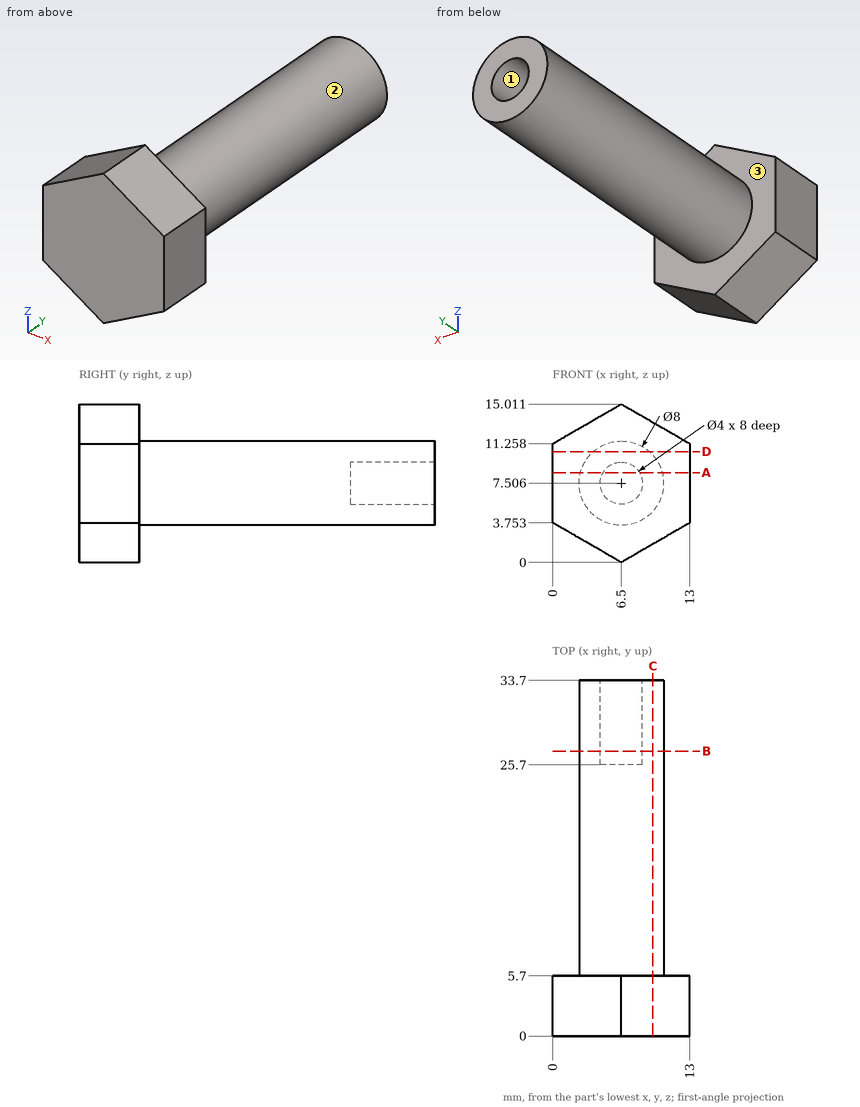
Could you check a few things on this drawing? It's one solid part, dimensions in mm from its lowest x, y, z. Coordinates: 2 decimals unless noted, no trailing zeros. Order: outer loops, then holes, each group sorted by start corner. A loop starts at its lowest first (then second) coordinate and runs counter-clockwise, first axis right, second up. Notation, with made-up numbers: (11.25, -32.5) - (26.25, -32.5) arc R23 ccw to (26.25, 0.5) - close; hole circle Ø9 at (56, -23.75). An arc over 180 degrees is marked (long way). Answer as a JSON object with one key per item and string values. Group by question number.
Q1. I need wall thicknesses on line 1 (X direction, y = 29.5, z = 7.5); line 2 (Y direction, x = 10.25, z = 10.25); line 3 (Z direction, x = 6.25, y = 23). Which ranges of each line are inside material? Lowest first, please. Write a range as from..to.
Q2. Imagine slicing it at A-A (z = 8.5). Please give me the cut outline in (x, y) (1 decimal).
Q3. Imagine slicing it at C-C (x = 9.5). Please give me the cut outline in (y, z), and give its area (3 significant figures).
Q4. Will these pins go through, and if not, where does the flat tip stop? P1, Ø1, axis at x = 3.5, y = 25, coming from the +Z side; P2, Ø1, axis at y = 13.5, z = 6.5, coming from the -X side; P3, Ø2, axis at x = 6, z = 8, coming from the +Y side.
Q5. Imagine slicing it at D-D (z = 10.5). Please give me the cut outline in (x, y), and give its area (3 significant figures).
Q6. Imagine slicing it at B-B (y = 27). Please give me the cut outline in (x, z) (1 decimal).
Q7. We'd pull the mould along Z, two halves only. Please class the marked faces 1, 2 and 3: +Z half, -Z half, draft (parallel to the pull), parting line (faces both ways), or undercut.
Determined:
{
 "1": {"line 1": "x = 2.5..4.5, 8.5..10.5", "line 2": "y = 0..5.7", "line 3": "z = 3.51..11.5"},
 "2": {"outline": "(0, 0) - (13, 0) - (13, 5.7) - (10.4, 5.7) - (10.4, 33.7) - (8.2, 33.7) - (8.2, 25.7) - (4.8, 25.7) - (4.8, 33.7) - (2.6, 33.7) - (2.6, 5.7) - (0, 5.7) - close"},
 "3": {"outline": "(0, 1.73) - (5.7, 1.73) - (5.7, 4.86) - (33.7, 4.86) - (33.7, 10.15) - (5.7, 10.15) - (5.7, 13.28) - (0, 13.28) - close", "area": "214 mm2"},
 "4": {"P1": "stops at z = 10.63", "P2": "stops at x = 2.53", "P3": "stops at y = 25.7"},
 "5": {"outline": "(0, 0) - (13, 0) - (13, 5.7) - (9.15, 5.7) - (9.15, 33.7) - (3.85, 33.7) - (3.85, 5.7) - (0, 5.7) - close", "area": "223 mm2"},
 "6": {"outline": "circle Ø8 at (6.5, 7.5); hole circle Ø4 at (6.5, 7.5)"},
 "7": {"face 1": "undercut", "face 2": "parting line", "face 3": "draft"}
}
